Here's the drawing with two shaded views (mm, measured from the low corner). I have some questions. A direction names the side the tool comes from. Give positions to 0.01 mm unless a question says otherwise; leave off trailing zeros. Write each loop counter-clockwise with the first axis right and the second up, starting at its lowest first coordinate (ties: lowest second). Pieces come first, ordered by that corner, then holes.
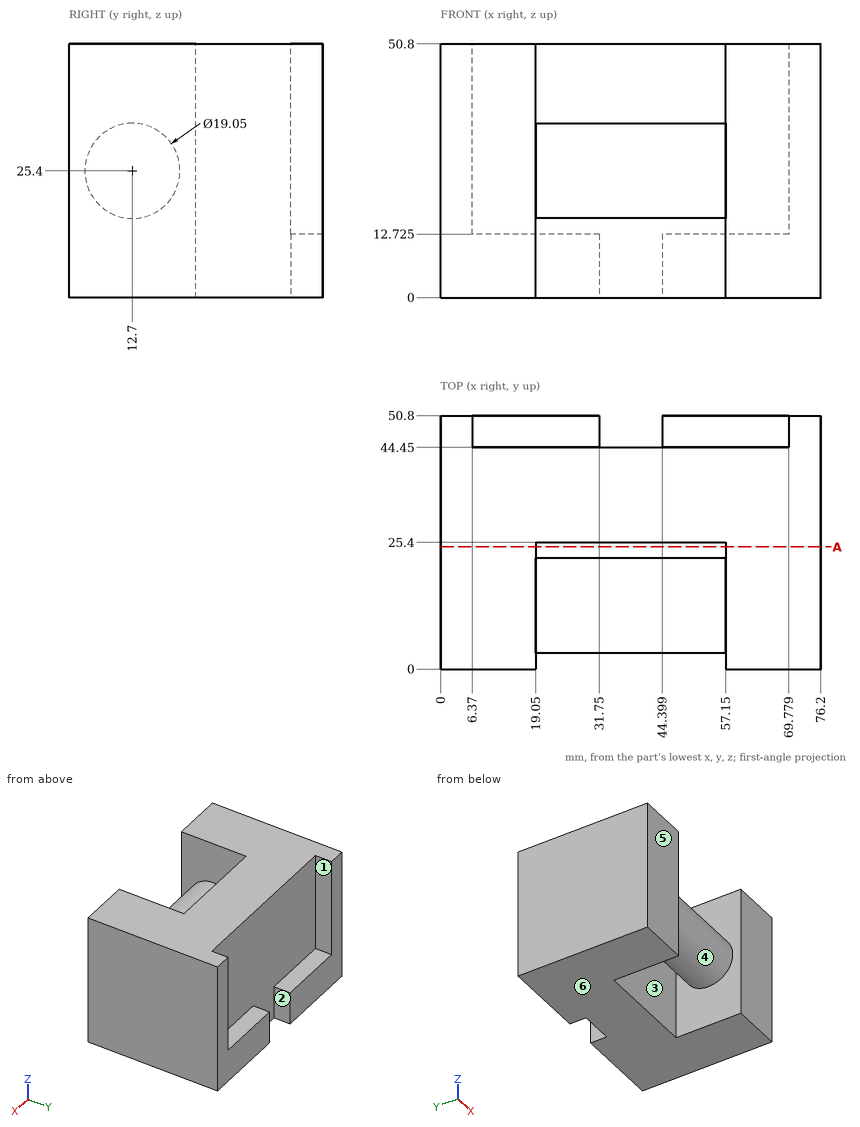
(1) If we mould it in two halves opening along Y, with no side actions, what happens to the marked faces 4, 5 and 6? For each: +Y half, -Y half, draft (parallel to the pull), parting line (faces both ways), or undercut.
Returned:
face 4: undercut
face 5: -Y half
face 6: draft
(2) For the marked faces 1, 2 and 3, which set-ups out of +Z, -Z, +X, -X, +Y, -Y let a thin tool reach every point of the face, with its end or its side?
Returned:
face 1: +Z, +Y
face 2: +Z, -Z, +Y
face 3: +Z, -Z
(3) Imagine slicing it at A-A, the plane y = 24.5. Write out the boundary of the cut face in (x, z).
Returned:
outline: (0, 0) - (19.05, 0) - (19.05, 50.8) - (0, 50.8) - close; (57.15, 0) - (76.2, 0) - (76.2, 50.8) - (57.15, 50.8) - close
(4) Will these pins go through, and if not, where does the flat tip stop? P1, Ø19, axis at x = 41, z = 33.5, coming from the -Y side (3 decimals); P2, Ø1.5, axis at x = 54.5, z = 28, coming from the +Y side; P3, Ø3, axis at x = 24.5, y = 48.5, coming from the +Z side (1 decimal).
Returned:
P1: stops at y = 3.175
P2: stops at y = 44.45
P3: stops at z = 12.7
(5) If I drill on L1, parallel to X at y = 9, z = 3.5; L2, parallel to Z at x = 10, y = 46.5 (1 decimal), over which ranges is the centre line in solid material (lowest first)?
Returned:
L1: x = 0 to 19.05, 57.15 to 76.2
L2: z = 0 to 12.7
